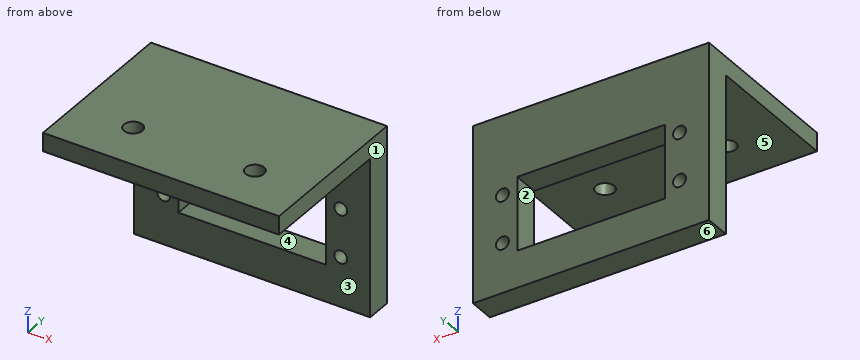
Autodesk Fusion 360 part; units mm, degrees
sketch "Sketch1" plane through (0, 0, 0) normal (0, 1, 0) x (1, 0, 0)
sketch "Sketch2" plane through (0, 0, 0) normal (0, 1, 0) x (1, 0, 0)
  line L0 (0, 0) -> (40, 0)
  line L1 (40, 0) -> (40, 20)
  line L2 (40, 20) -> (0, 20)
  line L3 (0, 20) -> (0, 0)
  line L4 (-12, -18) -> (52, -18)
  line L5 (52, -18) -> (52, 30)
  line L6 (52, 30) -> (-12, 30)
  line L7 (-12, 30) -> (-12, -18)
  line L8 (44, 20) -> (44, 16.5) construction
  line L9 (44, 0) -> (44, 3.5) construction
  line L10 (40, 16.5) -> (44, 16.5) construction
  line L11 (40, 3.5) -> (44, 3.5) construction
  circle A0 centre (44, 16.5) radius 1.75
  circle A1 centre (44, 3.5) radius 1.75
  line L12 (-4, 20) -> (-4, 16.5) construction
  line L13 (0, 16.5) -> (-4, 16.5) construction
  line L14 (0, 3.5142) -> (-4, 3.5126) construction
  line L15 (-4, 0.0126) -> (-4, 3.5126) construction
  circle A2 centre (-4, 16.5) radius 1.75
  circle A3 centre (-4, 3.5126) radius 1.75
  dimension "d1" = 40
  dimension "d2" = 20
  dimension "d8" = 18
  dimension "d9" = 10
  dimension "d10" = 3.5
  dimension "d11" = 3.5
  dimension "d12" = 4
  dimension "d13" = 4
  dimension "d14" = 3.5
  dimension "d15" = 3.5
  dimension "d16" = 3.5
  dimension "d17" = 4
  dimension "d18" = 4
  dimension "d19" = 3.5
  dimension "d20" = 3.5
  dimension "d21" = 3.5
  dimension "d22" = 12
  dimension "d23" = 12
extrude "Extrude1" add sketch "Sketch2" along normal blind 7
sketch "Sketch3" plane through (0, 7, 0) normal (0, 1, 0) x (-1, 0, 0)
  circle A0 centre (4, -3.5126) radius 1.75
  circle A1 centre (-44, -16.5) radius 1.75
  circle A2 centre (4, -16.5) radius 1.75
  circle A3 centre (-44, -3.5) radius 1.75
  line L0 (0, 0) -> (0, -20)
  line L1 (0, -20) -> (-40, -20)
  line L2 (-40, -20) -> (-40, 0)
  line L3 (-40, 0) -> (0, 0)
  line L4 (12, -30) -> (12, 18)
  line L5 (12, 18) -> (-52, 18)
  line L6 (-52, 18) -> (-52, -30)
  line L7 (-52, -30) -> (12, -30)
  line L8 (12, 18) -> (-52, 18)
  line L9 (-52, 18) -> (-52, 13)
  line L10 (-52, 13) -> (12, 13)
  line L11 (12, 13) -> (12, 18)
  dimension "d26" = 5
extrude "Extrude2" add sketch "Sketch3" against normal blind 45 contours L4 L5 L6 L8 L9 L10 L11
sketch "Sketch4" plane through (0, 0, 13) normal (0, 0, -1) x (-1, 0, 0)
  line L0 (12, 0) -> (-52, 0)
  line L1 (-52, 0) -> (-52, -38)
  line L2 (-52, -38) -> (12, -38)
  line L3 (12, -38) -> (12, 0)
  circle A0 centre (-37, -25) radius 2.5
  circle A1 centre (-4, -25) radius 2.5
  dimension "d29" = 5
  dimension "d30" = 5
extrude "Extrude3" cut sketch "Sketch4" against normal blind 10 contours A0 | A1
Could you check a few things on this model? Use its own coordinates, in mm. Face numbers are marked on the shaded views. A direction names the side the tool comes from. Coordinates: 2 decimals unless noted, no trailing zeros. Loops run counter-clockwise (first coordinate to the right, second up) from the corner with the lowest first, then second, coordinate; pieces in that order, holes last. Notation, with made-up numbers: (39.5, 21) -> (65.5, 21) arc R17 ccw to (65.5, 54) -> close; hole circle Ø3 at (2, 27.5). An arc over 180 degrees is marked (long way). Answer in a Markdown table with one row per item.
(1) If I drill on probe 1 along X at (y, z) = (4.5, -3.5); probe 2 along Z at (x, y) = (-4, 5); probe 3 along X at (y, z) = (0.5, -11), over which ranges is the centre line in solid material (lowest first)?
Results found:
| item | result |
|---|---|
| probe 1 | x = -12 to -5.75, -2.25 to 0, 40 to 42.25, 45.75 to 52 |
| probe 2 | z = -30 to -18.25, -14.75 to -5.26, -1.76 to 18 |
| probe 3 | x = -12 to 0, 40 to 52 |
(2) Imagine slicing it at B-B (y = -25). List the corners of the cut face in (x, z) for me, plus the area to 3 significant figures.
Results found:
| item | result |
|---|---|
| outline | (-12, 13) -> (1.5, 13) -> (1.5, 18) -> (-12, 18) -> close; (6.5, 13) -> (34.5, 13) -> (34.5, 18) -> (6.5, 18) -> close; (39.5, 13) -> (52, 13) -> (52, 18) -> (39.5, 18) -> close |
| area | 270 mm^2 |
(3) For the marked faces 4, 5 and 6, which set-ups out of +Z, -Z, +X, -X, +Y, -Y let a thin tool reach every point of the face, with its end or its side?
Results found:
| item | result |
|---|---|
| face 4 | +Y, -Y |
| face 5 | -Z, +X, -X, -Y |
| face 6 | -Z, +X, -X, +Y, -Y |
(4) Thinking about a two-plate mould opening in X: for the marked faces 1, 2 and 3, which applies, released by +X, released by -X, zero draft, split by the parting line, or undercut?
Results found:
| item | result |
|---|---|
| face 1 | released by +X |
| face 2 | undercut |
| face 3 | zero draft |
(5) Imagine slicing it at C-C (x = 8). List the corners of the cut face in (y, z) for me, plus the area to 3 significant figures.
Results found:
| item | result |
|---|---|
| outline | (-38, 13) -> (0, 13) -> (0, 0) -> (7, 0) -> (7, 18) -> (-38, 18) -> close; (0, -30) -> (7, -30) -> (7, -20) -> (0, -20) -> close |
| area | 386 mm^2 |
(6) Imagine slicing it at D-D (x = 44). List the corners of the cut face in (y, z) for me.
Results found:
| item | result |
|---|---|
| outline | (-38, 13) -> (0, 13) -> (0, -1.75) -> (7, -1.75) -> (7, 18) -> (-38, 18) -> close; (0, -30) -> (7, -30) -> (7, -18.25) -> (0, -18.25) -> close; (0, -14.75) -> (7, -14.75) -> (7, -5.25) -> (0, -5.25) -> close |
(7) Will these pins go through, and if not, where does the flat tip stop? pin 1 Ø2 at (x, y) = (15.5, -17) entering from -Z; pin 2 Ø1 at (x, z) = (28, 5.5) entering from -Y.
Results found:
| item | result |
|---|---|
| pin 1 | stops at z = 13 |
| pin 2 | stops at y = 0 |
(8) Imagine slicing it at A-A (z = -16.5). List the corners of the cut face in (x, y) for me, plus the area to 3 significant figures.
Results found:
| item | result |
|---|---|
| outline | (-12, 0) -> (-5.75, 0) -> (-5.75, 7) -> (-12, 7) -> close; (-2.25, 0) -> (0, 0) -> (0, 7) -> (-2.25, 7) -> close; (40, 0) -> (42.25, 0) -> (42.25, 7) -> (40, 7) -> close; (45.75, 0) -> (52, 0) -> (52, 7) -> (45.75, 7) -> close |
| area | 119 mm^2 |
